For this review, use the dimensioned drawing (mm, ordinates from the lowest corner) and the shaded views. Give positions to 0.01 mm unless a question says otherwise; leave off trailing zeros. Order: outer loops, then holes, each group sorted by start corner. A loop starts at its lowest first (then second) coordinate and runs counter-clockwise, first axis right, second up.
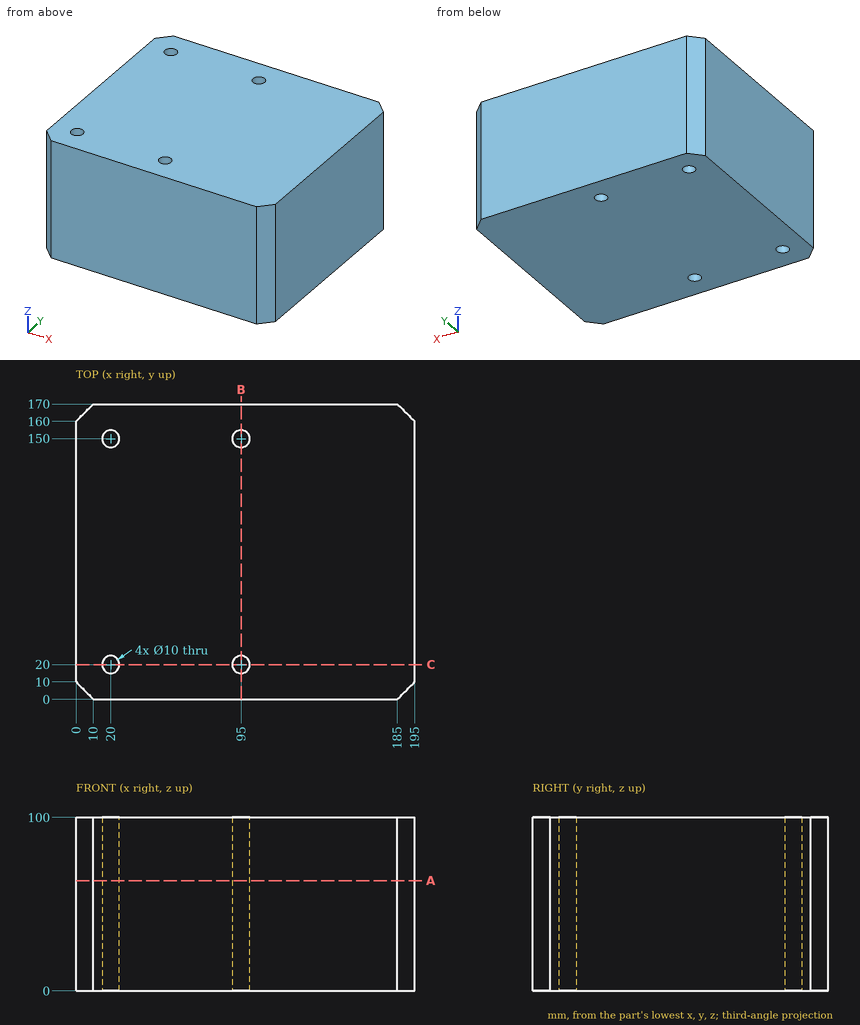
1. Take a section at A-A (z = 63.5). State the section outline as (x, y) points.
Recorded:
outline: (0, 10) - (10, 0) - (185, 0) - (195, 10) - (195, 160) - (185, 170) - (10, 170) - (0, 160) - close; hole circle Ø10 at (20, 20); hole circle Ø10 at (20, 150); hole circle Ø10 at (95, 20); hole circle Ø10 at (95, 150)
2. Take a section at B-B (x = 95). State the section outline as (y, z) points.
Recorded:
outline: (0, 0) - (15, 0) - (15, 100) - (0, 100) - close; (25, 0) - (145, 0) - (145, 100) - (25, 100) - close; (155, 0) - (170, 0) - (170, 100) - (155, 100) - close
3. Take a section at C-C (y = 20). State the section outline as (x, z) points.
Recorded:
outline: (0, 0) - (15, 0) - (15, 100) - (0, 100) - close; (25, 0) - (90, 0) - (90, 100) - (25, 100) - close; (100, 0) - (195, 0) - (195, 100) - (100, 100) - close
4. For line 1 along X through (y, z) = (150, 31); line 2 along Y through (x, z) = (95, 53.5); line 3 along X through (y, z) = (151.5, 28.5), list the stretches that pass through material, from the lowest coordinate up.
Recorded:
line 1: x = 0 to 15, 25 to 90, 100 to 195
line 2: y = 0 to 15, 25 to 145, 155 to 170
line 3: x = 0 to 15.23, 24.77 to 90.23, 99.77 to 195
